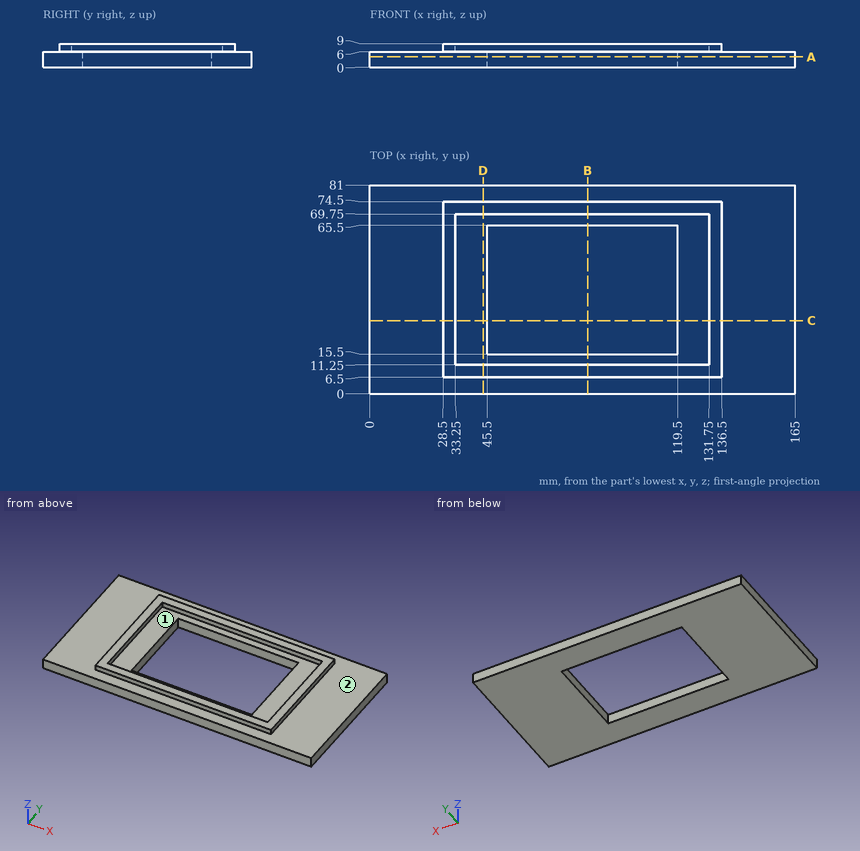
Source: three-view drawing plus pictorial views. Frame: mm from the lowest corner of the part. Give positions to 0.01 mm unless a question says otherwise; leave off trailing zeros. Order: outer loops, then holes, each group sorted by start corner. A loop starts at its lowest first (then second) coordinate and runs counter-clockwise, first axis right, second up. Notation, with made-up numbers: (61.5, -23) -> (102.5, -23) arc R7 ccw to (102.5, -10) -> close; hole circle Ø4 at (-2.75, 83). An arc over 180 degrees is marked (long way). Write each question's results on one line, items separated by ' | '. Start each with the question number.
Item 1: Line query: line 1 (Y direction, x = 82.5, z = 1); line 2 (X direction, y = 48, z = 4.5); line 3 (Y direction, x = 70, z = 6.5). Output: solid intervals per line, ascending.
Item 2: Cut plane B-B on x = 84.5. Return the cut outline in (y, z), then the cut area to 4 significant figures.
Item 3: Contact query for flat-ended pins moving along their axis: P1, Ø1.5, axis at x = 62.5, z = 7, coming from the -Y side; P2, Ø2.5, axis at x = 109, z = 7, coming from the +Y side; P3, Ø0.9, axis at y = 30.5, z = 7, coming from the +X side; P4, Ø0.9, axis at y = 46, z = 7, coming from the -X side. Output: stop coordinate, or through.
Item 4: Mould query, pull axis X, two halves, no side actions, for the marked faces 1 and 2. Classes: pulls with the +X half, pulls with the -X half, needs draft (parallel to the pull), parting line crosses it, or undercut.
Item 5: Cut plane D-D on x = 44. Return the cut outline in (y, z), then the cut area to 4 significant figures.
Item 6: Cut plane A-A on z = 4. Return the cut outline in (x, y).
Item 7: Cut plane C-C on y = 28.5. Return the cut outline in (x, z).
Established:
1) line 1: 0 to 15.5, 65.5 to 81 | line 2: 0 to 45.5, 119.5 to 165 | line 3: 6.5 to 11.25, 69.75 to 74.5
2) outline: (0, 0) -> (15.5, 0) -> (15.5, 6) -> (11.25, 6) -> (11.25, 9) -> (6.5, 9) -> (6.5, 6) -> (0, 6) -> close; (65.5, 0) -> (81, 0) -> (81, 6) -> (74.5, 6) -> (74.5, 9) -> (69.75, 9) -> (69.75, 6) -> (65.5, 6) -> close | area: 214.5 mm^2
3) P1: y = 6.5 | P2: y = 81 | P3: x = 136.5 | P4: x = 28.5
4) face 1: undercut | face 2: needs draft
5) outline: (0, 0) -> (81, 0) -> (81, 6) -> (74.5, 6) -> (74.5, 9) -> (69.75, 9) -> (69.75, 6) -> (11.25, 6) -> (11.25, 9) -> (6.5, 9) -> (6.5, 6) -> (0, 6) -> close | area: 514.5 mm^2
6) outline: (0, 0) -> (165, 0) -> (165, 81) -> (0, 81) -> close; hole (45.5, 15.5) -> (119.5, 15.5) -> (119.5, 65.5) -> (45.5, 65.5) -> close
7) outline: (0, 0) -> (45.5, 0) -> (45.5, 6) -> (33.25, 6) -> (33.25, 9) -> (28.5, 9) -> (28.5, 6) -> (0, 6) -> close; (119.5, 0) -> (165, 0) -> (165, 6) -> (136.5, 6) -> (136.5, 9) -> (131.75, 9) -> (131.75, 6) -> (119.5, 6) -> close
